Autodesk Inventor part; units mm, degrees
ref_plane "YZ Plane" through (0, 0, 0) normal (1, 0, 0) x (0, 1, 0)
ref_plane "XZ Plane" through (0, 0, 0) normal (0, 1, 0) x (-1, 0, 0)
ref_plane "XY Plane" through (0, 0, 0) normal (0, 0, 1) x (1, 0, 0)
sketch "Sketch1" plane through (0, 0, 0) normal (0, 1, 0) x (-1, 0, 0)
  line L0 (0, 0) -> (148, 0)
  line L1 (148, 0) -> (148, -229)
  line L2 (148, -229) -> (0, -229)
  line L3 (0, -229) -> (0, 0)
  line L4 (0, 0) -> (10, 0) construction
  line L5 (10, 0) -> (10, -51) construction
  circle A0 centre (10, -51) radius 8
  line L6 (10, -59) -> (0, -59)
  line L7 (10, -43) -> (0, -43)
  line L8 (10, -51) -> (10, -177) construction
  circle A1 centre (10, -177) radius 8
  line L9 (10, -169) -> (0, -169)
  line L10 (10, -185) -> (0, -185)
  line L11 (148, 0) -> (138, 0) construction
  line L12 (138, 0) -> (138, -51) construction
  circle A2 centre (138, -51) radius 8
  line L13 (138, -59) -> (148, -59)
  line L14 (138, -43) -> (148, -43)
  line L15 (138, -51) -> (138, -177) construction
  circle A3 centre (138, -177) radius 8
  line L16 (138, -185) -> (148, -185)
  line L17 (138, -169) -> (148, -169)
  dimension "d0" = 148
  dimension "d1" = 229
  dimension "d2" = 10
  dimension "d3" = 51
  dimension "d4" = 16
  dimension "d5" = 126
  dimension "d6" = 16
  dimension "d7" = 10
  dimension "d8" = 51
  dimension "d9" = 16
extrude "Extrusion1" add sketch "Sketch1" along normal blind 3 contours L0 L1 L14 A2 L13 L17 A3 L16 L2 L3 L10 A1 L9 L6 A0 L7
properties part number "heater"
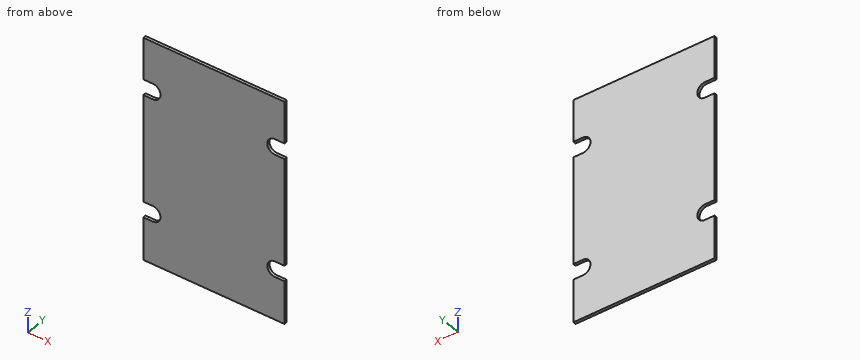
Work out the finished part from the listing and answer in its coordinate system (mm). Coordinates: 2 decimals unless noted, no trailing zeros. Loops run counter-clockwise (first coordinate to the right, second up) from the corner with the lowest first, then second, coordinate; pieces in that order, holes last. Notation, with made-up numbers: M 5,-13 L 11,-13 A20 ccw 11,24 Z; hole C 37,9 d2. An arc over 180 degrees is marked long. Answer in a Markdown table with one row per item. Add a question column.
1. Consider L1, parallel to Z at x = -7, y = 0.3; L2, parallel to Z at x = -134.5, y = 1.35; L3, parallel to X at y = 2.7, z = -53. Determine where each line is inside the solid, lowest interval first.
2. Find section B-B, the plane z = -51. Write down the section's boundary in (x, y), then the cut area to 3 significant figures.
3. Find section A-A, the plane y = 1.8. Write down the section's boundary in (x, z), then the cut area to 3 significant figures.
Reported:
| question | item | result |
|---|---|---|
| 1 | L1 | z = -229 to -185, -169 to -59, -43 to 0 |
| 1 | L2 | z = -229 to -184.19, -169.81 to -58.19, -43.81 to 0 |
| 1 | L3 | x = -130.25 to -17.75 |
| 2 | outline | M -130,0 L -18,0 L -18,3 L -130,3 Z |
| 2 | area | 336 mm^2 |
| 3 | outline | M -148,-229 L 0,-229 L 0,-185 L -10,-185 A8 cw -10,-169 L 0,-169 L 0,-59 L -10,-59 A8 cw -10,-43 L 0,-43 L 0,0 L -148,0 L -148,-43 L -138,-43 A8 cw -138,-59 L -148,-59 L -148,-169 L -138,-169 A8 cw -138,-185 L -148,-185 Z |
| 3 | area | 32,800 mm^2 |
